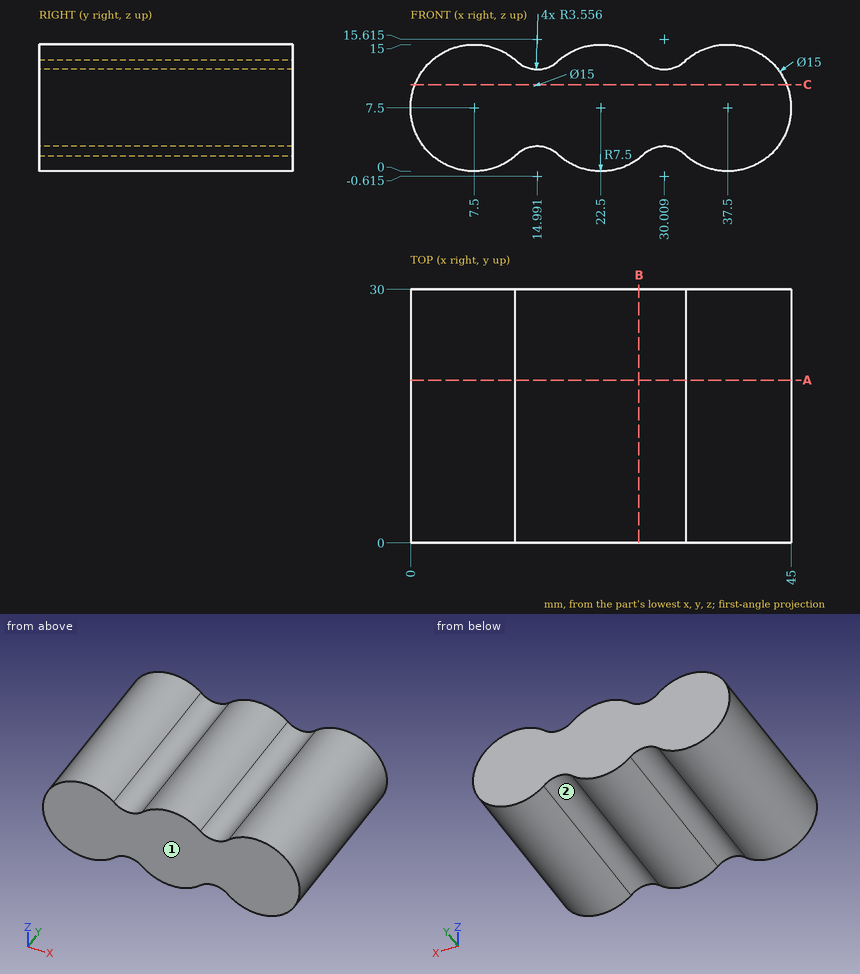
Part print with two shaded views. Sizes in mm from the minimum x, y, z corner. Round coordinates to 2 decimals unless told otherwise and drop trailing zeros. Write each loop counter-clockwise with the first axis right and the second up, starting at its lowest first coordinate (ties: lowest second). Pieces come first, ordered by that corner, then holes. Notation, with made-up numbers: (-25.75, -28) -> (16.25, -28) arc R20 cw to (16.25, 9) -> close; hole circle Ø2 at (-7.75, -18.5). An arc over 180 degrees is marked (long way). Use one line per item in the form item = value.
Q1. Band-saw the part on B-B, the plane x = 27. Write the cut outline in (y, z).
Conclusion:
outline = (0, 1.5) -> (30, 1.5) -> (30, 13.5) -> (0, 13.5) -> close
Q2. Two-plate mould, pull along X, no slides. Class the marked faces 1 and 2: released by +X, released by -X, zero draft, split by the parting line, or undercut.
Conclusion:
face_1 = zero draft
face_2 = undercut
Q3. Drop flat-ended pins along their axis: P1, Ø2, axis at y = 6, z = 13.5, coming from the -X side; P2, Ø1.5, axis at x = 36, z = 4, coming from the -Y side; P3, Ø1.5, axis at y = 12, z = 11.5, coming from the +X side; P4, Ø4, axis at x = 13, y = 19.5, coming from the -Z side. Give the stop position or say it passes through.
Conclusion:
P1 = 1.91
P2 = 0
P3 = 44.26
P4 = 0.87
Q4. Band-saw the part on C-C, the plane z = 10.25. Write the cut outline in (x, y).
Conclusion:
outline = (0.52, 0) -> (44.48, 0) -> (44.48, 30) -> (0.52, 30) -> close
Q5. Band-saw the part on A-A, the plane y = 19.25. Write the cut outline in (x, z) (1 decimal), then the cut area to 3 significant figures.
Conclusion:
outline = (12.4, 1.8) arc R3.6 cw to (17.4, 2) arc R7.5 ccw to (27.6, 2) arc R3.6 cw to (32.6, 1.8) arc R7.5 ccw (long way) to (32.6, 13.2) arc R3.6 cw to (27.6, 13) arc R7.5 ccw to (17.4, 13) arc R3.6 cw to (12.4, 13.2) arc R7.5 ccw (long way) to start
area = 550 mm²
Q6. Drill centre lines: L1, parallel to X at y = 6.5, z = 12.75 (1 decimal); L2, parallel to X at y = 9.5, z = 2.5 (1 decimal); L3, parallel to Z at x = 31, y = 8.5. Where is each one in solid material? Low to high.
Conclusion:
L1 = 2.1 to 12.9, 17.1 to 27.9, 32.1 to 42.9
L2 = 1.9 to 13.3, 16.7 to 28.3, 31.7 to 43.1
L3 = 2.8 to 12.2
